Geometry: final body of the model. Coordinates: model frame, mm. A direction names the side the tool comes from. Give positions to 0.01 mm unless a question says otherwise; leave off trailing zeros. Write each loop counter-clockwise with the first axis right and the second up, starting at its lowest first coordinate (ties: lowest second). Pieces come first, ordered by that corner, then holes. Notation, with made-up numbers: (55.25, 54.5) -> (62.25, 54.5) arc R12 ccw to (62.25, 65.5) -> close; hole circle Ø8 at (-33, -5). An arc over 180 degrees is marked (long way). Answer in a Markdown table with one row per item. Add a question column.
Item 1: Section query B-B on z = 5.5. Output: boundary loops of the cut face in (x, y), plus the area to 3 significant figures.
Item 2: Access query for faces 4 (the flat face through (75.07, 29.37, 0.56)), 5 (the cylindrical face through (-6, 4, -38)), 6 (the cylindrical face through (96, -6, 38)), 7 (the cylindrical face through (96, -6, -38)). Directions: +Z, -Z, +X, -X, +Y, -Y. A direction counts if a zero-diameter tool reaches every point of the face in a straight line with its end or side. Return the directions, or none.
Item 3: First-contact query: P1, Ø1.6, axis at x = -6, z = -3, coming from the +Y side; P2, Ø4, axis at y = 2, z = 11, coming from the +X side; P3, Ø2, axis at y = 61, z = 24, coming from the -X side. Flat tips, straight axial feed; report the tip coordinate or a pass-through.
Item 4: Section query C-C on x = 8. Output: boundary loops of the cut face in (y, z), plus the area to 3 significant figures.
Item 5: Section query A-A on y = 62.5. Output: boundary loops of the cut face in (x, z), plus the area to 3 significant figures.
Item 6: Draft query along X for faces 1 (the cylindrical face through (-6, 4, 38)), 2 (the cylindrical face through (-1.32, -5.34, 0.56)), 3 (the flat face through (77.165, 28.735, 0.56)). Return one class per face: +X half, -X half, draft (parallel to the pull), parting line (faces both ways), or undercut.
Item 7: Material intervals for probe 1 along Y at (x, z) = (0.5, 35); probe 2 along X at (y, z) = (65.5, -24.5); probe 3 along X at (y, z) = (28, 16), sorted ascending. Write a range as from..to.
```python
from build123d import *

# Parameters (mm, degrees)
F1_DEPTH    = 40
F2_T1_DEPTH = 14
F2_T3_DEPTH = 26.7295341336


# Not quite as in the source:
# - a fillet or chamfer that OpenCascade refuses, or shapes differently, is made with other operations: its cross-section is extruded or revolved along the edge and cut away or added


with BuildPart() as f1:
    # F0 (on Top) → F1 (new body, symmetric)
    with BuildSketch(Plane.XY):
        with BuildLine():
            Line((-7, 5), (-7, 0))
            ThreePointArc((-7, 0), (-1.8031925829, -6.7637634871), (6.0709990026, -3.484676615))
            Line((6.0709990026, -3.484676615), (45.2299293551, 64.7379601975))
            ThreePointArc((45.2299293551, 64.7379601975), (50, 67.5), (54.7700706449, 64.7379601975))
            Line((54.7700706449, 64.7379601975), (95.9467521433, -7))
            Line((95.9467521433, -7), (97.6762862769, -7))
            Line((97.6762862769, -7), (56.0709990026, 65.484676615))
            ThreePointArc((56.0709990026, 65.484676615), (50, 69), (43.9290009974, 65.484676615))
            Line((43.9290009974, 65.484676615), (4.7700706449, -2.7379601975))
            ThreePointArc((4.7700706449, -2.7379601975), (-1.4167941723, -5.314385597), (-5.5, 0))
            Line((-5.5, 0), (-5.5, 5))
            Line((-5.5, 5), (-7, 5))
        make_face()
    extrude(amount=F1_DEPTH, both=True)

    # F2: fillet of radius 5 on 4 edges, made by hand

    # F2_s2 → F2_t1 (cut)
    with BuildSketch(Plane.YZ.offset(-19.5)):
        with BuildLine():
            ThreePointArc((5, 35), (3.5355339059, 38.5355339059), (0, 40))
            Line((0, 40), (5, 40))
            Line((5, 40), (5, 35))
        make_face()
        with BuildLine():
            ThreePointArc((5, -35), (3.5355339059, -38.5355339059), (0, -40))
            Line((0, -40), (5, -40))
            Line((5, -40), (5, -35))
        make_face()
    extrude(amount=F2_T1_DEPTH, mode=Mode.SUBTRACT)

    # F2_s4 → F2_t3 (cut)
    with BuildSketch(Plane.YZ.offset(83.4467521433)):
        with BuildLine():
            ThreePointArc((-7, 35), (-5.5355339059, 38.5355339059), (-2, 40))
            Line((-2, 40), (-7, 40))
            Line((-7, 40), (-7, 35))
        make_face()
        with BuildLine():
            ThreePointArc((-7, -35), (-5.5355339059, -38.5355339059), (-2, -40))
            Line((-2, -40), (-7, -40))
            Line((-7, -40), (-7, -35))
        make_face()
    extrude(amount=F2_T3_DEPTH, mode=Mode.SUBTRACT)


solid = f1.part
```
Findings below:
| question | item | result |
|---|---|---|
| 1 | outline | (-7, 0) arc R7 ccw to (6.07, -3.48) -> (45.23, 64.74) arc R5.5 cw to (54.77, 64.74) -> (95.95, -7) -> (97.68, -7) -> (56.07, 65.48) arc R7 ccw to (43.93, 65.48) -> (4.77, -2.74) arc R5.5 cw to (-5.5, 0) -> (-5.5, 5) -> (-7, 5) -> close |
| 1 | area | 294 mm^2 |
| 2 | face 4 | +Z, -Z, -Y |
| 2 | face 5 | -Z, -X, +Y |
| 2 | face 6 | +Z, +X, -Y |
| 2 | face 7 | -Z, +X, -Y |
| 3 | P1 | stops at y = 5 |
| 3 | P2 | stops at x = 93.66 |
| 3 | P3 | stops at x = 40.78 |
| 4 | outline | (-0.12, -40) -> (2.89, -40) -> (2.89, 40) -> (-0.12, 40) -> close |
| 4 | area | 241 mm^2 |
| 5 | outline | (42.22, -40) -> (43.95, -40) -> (43.95, 40) -> (42.22, 40) -> close; (56.05, -40) -> (57.78, -40) -> (57.78, 40) -> (56.05, 40) -> close |
| 5 | area | 277 mm^2 |
| 6 | face 1 | draft |
| 6 | face 2 | undercut |
| 6 | face 3 | +X half |
| 7 | probe 1 | y = -6.98..-5.48 |
| 7 | probe 2 | x = 43.94..45.76, 54.24..56.06 |
| 7 | probe 3 | x = 22.41..24.14, 75.86..77.59 |
